from build123d import *

# Parameters (mm, degrees)
SZKIC2_W                    = 14.5
SZKIC2_H                    = 5.1
DODANIE_WYCI_GNI_CIE1_DEPTH = 11.8
SZKIC3_R                    = 2.5
SZKIC3_R_2                  = 2
DODANIE_WYCI_GNI_CIE2_DEPTH = 0.5
SZKIC4_R                    = 2
DODANIE_WYCI_GNI_CIE3_DEPTH = 1
SZKIC5_R                    = 1.25
DODANIE_WYCI_GNI_CIE4_DEPTH = 0.8
SZKIC6_R                    = 0.65
DODANIE_WYCI_GNI_CIE5_DEPTH = 1
ZAOKR_GLENIE1_R             = 0.2
DODANIE_WYCI_GNI_CIE7_DEPTH = 5.1
SZKIC11_W                   = 0.45
SZKIC11_H                   = 5.401514826
WYTNIJ_WYCI_GNI_CIE2_DEPTH  = 23.306334437
WYTNIJ_WYCI_GNI_CIE3_DEPTH  = 0.778786
WYTNIJ_WYCI_GNI_CIE4_DEPTH  = 5
ZAOKR_GLENIE2_R             = 0.1
SZKIC14_R                   = 0.69
DODANIE_WYCI_GNI_CIE8_DEPTH = 5
SZKIC15_R                   = 0.4
DODANIE_WYCI_GNI_CIE9_DEPTH = 1
ZAOKR_GLENIE3_R             = 0.1


with BuildPart() as part:
    # Szkic2 → Dodanie-wyciągnięcie1 (new body)
    with BuildSketch(Plane(origin=(0, 0, 0), x_dir=(1, 0, 0), z_dir=(0, 1, 0))):
        Rectangle(SZKIC2_W, SZKIC2_H)
    extrude(amount=DODANIE_WYCI_GNI_CIE1_DEPTH)

    # Szkic3 → Dodanie-wyciągnięcie2 (add)
    with BuildSketch(Plane(origin=(0, 11.8, 0), x_dir=(1, 0, 0), z_dir=(0, 1, 0))):
        with Locations(Location((-4.75, 0, 0), (0, 0, 180))):
            Circle(SZKIC3_R)
        with Locations(Location((-4.75, 0, 0), (0, 0, 270))):
            Circle(SZKIC3_R_2, mode=Mode.SUBTRACT)
    extrude(amount=DODANIE_WYCI_GNI_CIE2_DEPTH)

    # Szkic4 → Dodanie-wyciągnięcie3 (add)
    with BuildSketch(Plane(origin=(0, 11.8, 0), x_dir=(1, 0, 0), z_dir=(0, 1, 0))):
        with Locations(Location((-4.75, 0, 0), (0, 0, 270))):
            Circle(SZKIC4_R)
    extrude(amount=DODANIE_WYCI_GNI_CIE3_DEPTH)

    # Szkic5 → Dodanie-wyciągnięcie4 (add)
    with BuildSketch(Plane(origin=(0, 12.8, 0), x_dir=(1, 0, 0), z_dir=(0, 1, 0))):
        with Locations(Location((-4.75, 0, 0), (0, 0, 270))):
            Circle(SZKIC5_R)
    extrude(amount=DODANIE_WYCI_GNI_CIE4_DEPTH)

    # Szkic6 → Dodanie-wyciągnięcie5 (add)
    with BuildSketch(Plane(origin=(0, 13.6, 0), x_dir=(1, 0, 0), z_dir=(0, 1, 0))):
        with Locations(Location((-4.75, 0, 0), (0, 0, 270))):
            Circle(SZKIC6_R)
    extrude(amount=DODANIE_WYCI_GNI_CIE5_DEPTH)

    # Zaokrąglenie1
    zaokr_glenie1_edges = [part.edges().sort_by_distance(p)[0] for p in [
        (-4.75, 12.8, -2),
        (-4.75, 13.6, -1.25),
    ]]
    fillet(zaokr_glenie1_edges, radius=ZAOKR_GLENIE1_R)

    # Szkic10 → Dodanie-wyciągnięcie7 (add)
    with BuildSketch(Plane.XY.offset(2.55)):
        with BuildLine():
            Line((6.75, 11.8), (6.75, 13.6))
            ThreePointArc((6.75, 13.6), (6.45374044, 14.20374044), (5.85, 14.5))
            Line((5.85, 14.5), (-8.25, 16.3))
            Line((-8.25, 16.3), (-8.262663189, 16.200805022))
            Line((-8.262663189, 16.200805022), (5.837336811, 14.400805022))
            ThreePointArc((5.837336811, 14.400805022), (6.378823054, 14.137558504), (6.65, 13.6))
            Line((6.65, 13.6), (6.65, 11.8))
            Line((6.65, 11.8), (6.75, 11.8))
        make_face()
    extrude(amount=-DODANIE_WYCI_GNI_CIE7_DEPTH)

    # Szkic11 → Wytnij-wyciągnięcie2 (cut, through all)
    with BuildSketch(Plane(origin=(6.75, 0, 0), x_dir=(0, 0, -1), z_dir=(1, 0, 0))):
        with Locations((-2.325, 15.000757413)):
            Rectangle(SZKIC11_W, SZKIC11_H)
        with Locations((2.325, 15.000757413)):
            Rectangle(SZKIC11_W, SZKIC11_H)
    extrude(amount=-WYTNIJ_WYCI_GNI_CIE2_DEPTH, mode=Mode.SUBTRACT)

    # Szkic12 → Wytnij-wyciągnięcie3 (cut)
    with BuildSketch(Plane(origin=(1.91518931, 15.002316258, 0), x_dir=(0.9919497796038491, -0.12663188675793827, 0), z_dir=(0.12663188675793827, 0.9919497796038491, 0))):
        with BuildLine():
            Line((-0.033256147, 0.1), (-0.033256147, -0.1))
            ThreePointArc((-0.033256147, -0.1), (0.142479784, -0.524264069), (0.566743853, -0.7))
            Line((0.566743853, -0.7), (3.966743853, -0.7))
            Line((3.966743853, -0.7), (8.34703338, -0.7))
            Line((8.34703338, -0.7), (8.34703338, 0.7))
            Line((8.34703338, 0.7), (3.966743853, 0.7))
            Line((3.966743853, 0.7), (0.566743853, 0.7))
            ThreePointArc((0.566743853, 0.7), (0.142479784, 0.524264069), (-0.033256147, 0.1))
        make_face()
    extrude(amount=-WYTNIJ_WYCI_GNI_CIE3_DEPTH, mode=Mode.SUBTRACT)

    # Szkic13 → Wytnij-wyciągnięcie4 (cut)
    with BuildSketch(Plane(origin=(6.75, 0, 0), x_dir=(0, 0, -1), z_dir=(1, 0, 0))):
        with BuildLine():
            Line((0.1, 12.3), (-0.1, 12.3))
            ThreePointArc((-0.1, 12.3), (-0.524264069, 12.475735931), (-0.7, 12.9))
            Line((-0.7, 12.9), (-0.7, 14.054695175))
            Line((-0.7, 14.054695175), (0.7, 14.054695175))
            Line((0.7, 14.054695175), (0.7, 12.9))
            ThreePointArc((0.7, 12.9), (0.524264069, 12.475735931), (0.1, 12.3))
        make_face()
    extrude(amount=-WYTNIJ_WYCI_GNI_CIE4_DEPTH, mode=Mode.SUBTRACT)

    # Zaokrąglenie2
    zaokr_glenie2_edges = [part.edges().sort_by_distance(p)[0] for p in [
        (-4.75, 14.6, -0.65),
    ]]
    fillet(zaokr_glenie2_edges, radius=ZAOKR_GLENIE2_R)

    # Szkic14 → Dodanie-wyciągnięcie8 (add)
    with BuildSketch(Plane(origin=(7.25, 0, 0), x_dir=(0, 0, -1), z_dir=(1, 0, 0))):
        with Locations(Location((0, 2.31, 0), (0, 0, 180))):
            Circle(SZKIC14_R)
        with Locations(Location((0.701480577, 1.095, 0), (0, 0, 180))):
            Circle(SZKIC14_R)
        with Locations(Location((-0.701480577, 1.095, 0), (0, 0, 180))):
            Circle(SZKIC14_R)
    extrude(amount=DODANIE_WYCI_GNI_CIE8_DEPTH)

    # Szkic15 → Dodanie-wyciągnięcie9 (add)
    with BuildSketch(Plane(origin=(12.25, 0, 0), x_dir=(0, 0, -1), z_dir=(1, 0, 0))):
        with Locations((0, 2.31)):
            Circle(SZKIC15_R)
        with Locations((0.701480577, 1.095)):
            Circle(SZKIC15_R)
        with Locations((-0.701480577, 1.095)):
            Circle(SZKIC15_R)
    extrude(amount=DODANIE_WYCI_GNI_CIE9_DEPTH)

    # Zaokrąglenie3
    zaokr_glenie3_edges = [part.edges().sort_by_distance(p)[0] for p in [
        (-8.256331594, 16.250402511, -2.1),
        (6.7, 12.3, -2.55),
        (-8.256331594, 16.250402511, 2.1),
        (6.7, 12.3, 2.55),
    ]]
    fillet(zaokr_glenie3_edges, radius=ZAOKR_GLENIE3_R)


solid = part.part
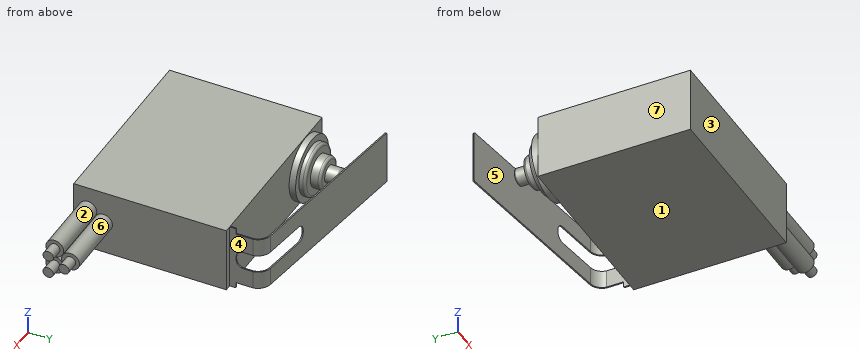
Model file for the job. Use its own axes, mm. Face numbers are marked on the shaded views. A direction names the side the tool comes from. Give positions to 0.01 mm unless a question says otherwise; leave off trailing zeros. Order: outer loops, then holes, each group sorted by start corner. A loop starts at its lowest first (then second) coordinate and runs counter-clockwise, first axis right, second up. Notation, with made-up numbers: (18.25, 85.5) - (56.25, 85.5) arc R12 ccw to (56.25, 90.5) - close; hole circle Ø2 at (36.5, 20). An arc over 180 degrees is marked (long way). Return JSON: item names as keys, results as strings.
1) Pull direction Z, two halves, no side cores. Call the marked faces 1, 2 and 3: pulls with the +Z half, pulls with the -Z half, needs draft (parallel to the pull), parting line crosses it, or undercut.
Geometry says:
{"face 1": "pulls with the -Z half", "face 2": "undercut", "face 3": "needs draft"}
2) Cut at D-D, the plane x = 10.5. Give the cut face in (y, z) (3 decimals), plus the area to 3 significant figures.
Geometry says:
{"outline": "circle Ø1.38 at (1.095, -0.701); circle Ø1.38 at (1.095, 0.701); circle Ø1.38 at (2.31, 0)", "area": "4.49 mm²"}
3) Cut at B-B, the plane y = 2.31. Give the cut face in (x, z), plus the area to 4 significant figures.
Geometry says:
{"outline": "(-7.25, -2.55) - (7.25, -2.55) - (7.25, -0.69) - (12.25, -0.69) - (12.25, -0.4) - (13.25, -0.4) - (13.25, 0.4) - (12.25, 0.4) - (12.25, 0.69) - (7.25, 0.69) - (7.25, 2.55) - (-7.25, 2.55) - close", "area": "81.65 mm²"}
4) Cut at A-A, the plane x = 1. Give the cut face in (y, z), plus the area to 3 significant figures.
Geometry says:
{"outline": "(0, -2.55) - (11.8, -2.55) - (11.8, 2.55) - (0, 2.55) - close; (15.02, -2.1) - (15.12, -2.1) - (15.12, 2.1) - (15.02, 2.1) - close", "area": "60.6 mm²"}
5) 3-axis set-ups, long thin cutter, end or side, ignore diameter. For the marked faces 4, 5, 6 and 7: which of +Z, -Z, +X, -X, +Y, -Y reach the whole face in a straight line?
Geometry says:
{"face 4": "+Z, -Z, +X, +Y", "face 5": "+Z, -Z, -X", "face 6": "+X", "face 7": "+Z, -Z, -X, -Y"}
6) Flat gauge pins, fed straight in: P1, Ø2, axis at x = 3.5, y = 14, coming from the +Z side; P2, Ø0.9, axis at y = 13, z = 0.5, coming from the +X side; P3, Ø2, axis at y = 1.5, z = 0, coming from the -X side; P4, Ø1, axis at x = 4, y = 13.5, coming from the -Z side. Where does each tip first touch, or does it go through?
Geometry says:
{"P1": "z = 2.1", "P2": "x = 6.75", "P3": "x = -7.25", "P4": "through"}
7) Probe line 1 (X direction, y = 4.75, z = 2.25); line 2 (X direction, y = 1, z = 0.35); line 3 (Y direction, x = 3, z = -0.05). List the from-to ranges inside material, lowest first. Write a range as from..to.
Geometry says:
{"line 1": "-7.25..7.25", "line 2": "-7.25..13.25", "line 3": "0..11.8"}
